Source: three-view drawing plus pictorial views. Frame: mm from the lowest corner of the part. Coordinates: 2 decimals unless noted, no trailing zeros. Loops run counter-clockwise (first coordinate to the right, second up) from the corner with the lowest first, then second, coordinate; pieces in that order, holes last. Notation, with made-up numbers: (43, 14.25) - (78, 14.25) arc R31 cw to (78, 42.25) - close; hole circle Ø1 at (36.5, 61). An arc over 180 degrees is marked (long way). Return JSON: item names as keys, results as strings.
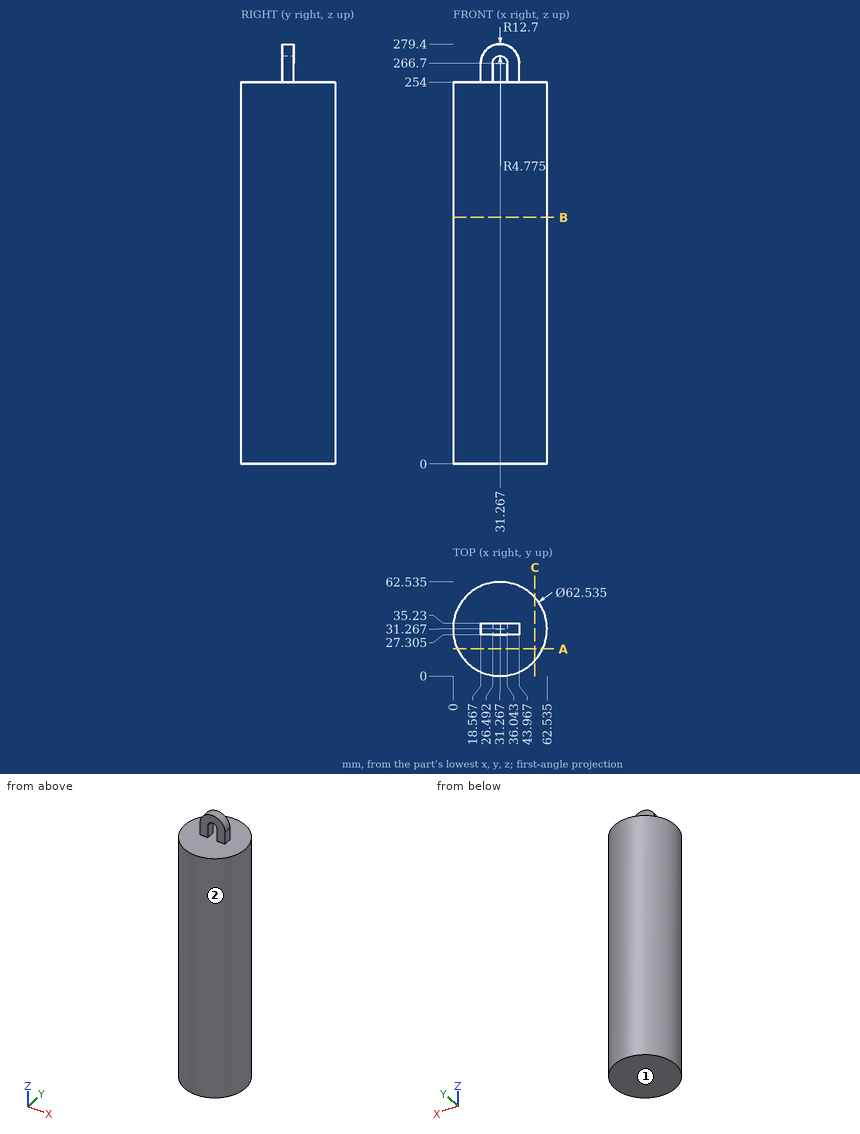
Item 1: Section query A-A, the plane y = 18. Return loops of the section in (x, z) (1 decimal).
Worked out:
{"outline": "(3, 0) - (59.6, 0) - (59.6, 254) - (3, 254) - close"}
Item 2: Mould query, pull axis Z, two halves, no side actions, for the marked faces 1 and 2. Classes: +Z half, -Z half, draft (parallel to the pull), parting line (faces both ways), or undercut.
Worked out:
{"face 1": "-Z half", "face 2": "draft"}
Item 3: Section query B-B, the plane z = 164. Return loops of the section in (x, y) (1 decimal).
Worked out:
{"outline": "circle Ø62.5 at (31.3, 31.3)"}
Item 4: Section query C-C, the plane x = 54.5. Return loops of the section in (y, z).
Worked out:
{"outline": "(10.34, 0) - (52.19, 0) - (52.19, 254) - (10.34, 254) - close"}
Item 5: Ray query, probe 1 along Z at (x, y) = (50, 30); probe 2 along X at (y, z) = (33, 259.5); probe 3 along Y at (x, z) = (31, 157.5). Return the intervals inside material, ascending. Write a range as from..to.
Worked out:
{"probe 1": "0..254", "probe 2": "18.57..26.49, 36.04..43.97", "probe 3": "0..62.53"}
Item 6: First-contact query: pin 1 Ø12 at (x, y) = (13.5, 20) entering from +Z; pin 2 Ø2.5 at (y, z) = (30.5, 262) entering from +X; pin 3 Ø1.5 at (x, z) = (37, 140.5) entering from +Y (1 decimal); pin 4 Ø5 at (x, y) = (36, 19.5) entering from -Z. Flat tips, straight axial feed; report the tip coordinate or a pass-through.
Worked out:
{"pin 1": "z = 254", "pin 2": "x = 43.97", "pin 3": "y = 62.1", "pin 4": "z = 0"}
